Check sheet for the modelled part. Datum: model origin and axes. Units: mm. Face numbers are marked on the shaded views. A direction names the side the tool comes from. Give positions to 0.01 mm unless a question says otherwise; leave off trailing zeros. Loops run counter-clockwise (first coordinate to the right, second up) from the corner with the lowest first, then second, coordinate; pieces in that order, holes last. Notation, with made-up numbers: (0.25, 10) -> (45.25, 10) arc R18 ccw to (45.25, 29) -> close; hole circle Ø4 at (-9.75, 33). An arc over 180 degrees is marked (long way). Answer as CSV lines item,"result". Start each with the question number.
(1) Gauge pin test, flat ends, axial feed: pin 1 Ø6 at (y, z) = (4, -1.5) entering from -X; pin 2 Ø4 at (y, z) = (15, -1.5) entering from +X; pin 3 Ø4 at (y, z) = (13, -6) entering from -X; pin 4 Ø3.5 at (x, y) = (0, 9.5) entering from +Z. Record the tip position at first contact, or that the pin passes through.
(2) Section check C-C on y = 7. Enter the section's corners in (x, z), plus the area to 3 significant figures.
(3) Material ranges on line 1 (Z direction, x = 0.5, y = 13.5); line 2 (Z direction, x = 0.5, y = 10.75); line 3 (X direction, y = 6.75, z = 0.5), recorded low to high. Write a range as from..to.
(4) Section check B-B on z = -1.25. Enter the section's corners in (x, y).
(5) Access from +Z, -Z, +X, -X, +Y, -Y to the whole of each face (thin tool, end or side, straight path). Record for the marked faces 1, 2 and 3.
from build123d import *

# Parameters (mm, degrees)
DODANIE_WYCI_GNI_CIE1_DEPTH = 1
SZKIC2_R                    = 3.5
DODANIE_WYCI_GNI_CIE2_DEPTH = 1
SZKIC3_R                    = 1.25
DODANIE_WYCI_GNI_CIE3_DEPTH = 10
ZAOKR_GLENIE1_R             = 1


with BuildPart() as part:
    # Szkic1 → Dodanie-wyciągnięcie1 (new body)
    with BuildSketch(Plane.XY):
        with BuildLine():
            Line((0.942427745, 2.655932737), (5.439447033, 15.32935073))
            ThreePointArc((5.439447033, 15.32935073), (5.485445584, 15.51205871), (5.496356907, 15.700151814))
            ThreePointArc((5.496356907, 15.700151814), (0, 21), (-5.496356907, 15.700151814))
            ThreePointArc((-5.496356907, 15.700151814), (-5.485445584, 15.51205871), (-5.439447033, 15.32935073))
            Line((-5.439447033, 15.32935073), (-0.942427745, 2.655932737))
            ThreePointArc((-0.942427745, 2.655932737), (0, 1.990342582), (0.942427745, 2.655932737))
        make_face()
    extrude(amount=DODANIE_WYCI_GNI_CIE1_DEPTH)

    # Szkic2 → Dodanie-wyciągnięcie2 (add)
    with BuildSketch(Plane.XY.offset(1)):
        with Locations((0, 15.5)):
            Circle(SZKIC2_R)
    extrude(amount=DODANIE_WYCI_GNI_CIE2_DEPTH)

    # Szkic3 → Dodanie-wyciągnięcie3 (add)
    with BuildSketch(Plane(origin=(0, 0, 0), x_dir=(-1, 0, 0), z_dir=(0, 0, -1))):
        with Locations((0, 15.5)):
            Circle(SZKIC3_R)
    extrude(amount=DODANIE_WYCI_GNI_CIE3_DEPTH)

    # Zaokrąglenie1
    zaokr_glenie1_edges = [part.edges().sort_by_distance(p)[0] for p in [
        (-3.5, 15.5, 2),
    ]]
    fillet(zaokr_glenie1_edges, radius=ZAOKR_GLENIE1_R - 0.0001)  # a hair under: the kernel refuses the full size


solid = part.part
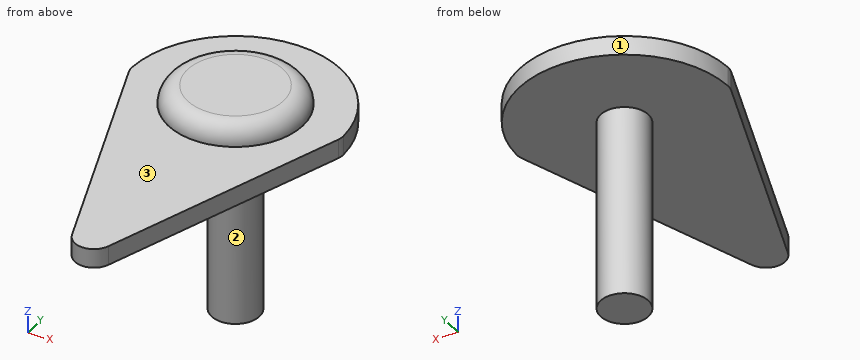
Working result:
1,pin 1,"stops at x = -2.34"
1,pin 2,"stops at x = 5.5"
1,pin 3,"stops at x = -1.15"
1,pin 4,"stops at z = 1"
2,outline,"(-2.48, 0) -> (2.48, 0) -> (2.48, 1) -> (-2.48, 1) -> close"
2,area,"4.97 mm^2"
3,line 1,"z = 0..2"
3,line 2,"z = 0..1"
3,line 3,"x = -2.4..2.4"
4,outline,"circle Ø2.5 at (0, 15.5)"
5,face 1,"+Z, -Z, +Y"
5,face 2,"-Z"
5,face 3,"+Z"
